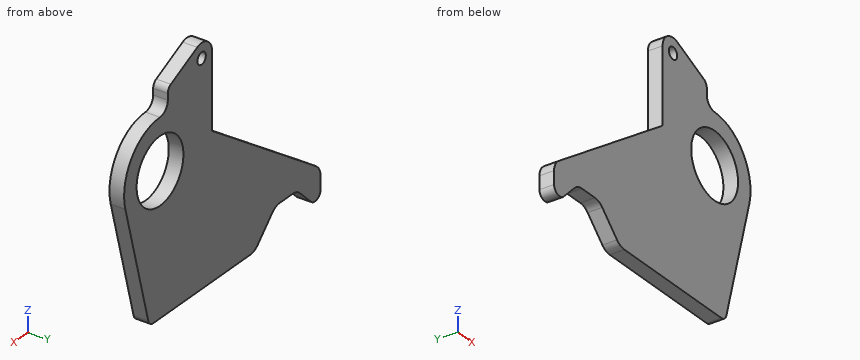
```python
from build123d import *

# Parameters (mm, degrees)
SKETCH1_R           = 2.5527
SKETCH1_R_2         = 14.2875
BOSS_EXTRUDE1_DEPTH = 6.35


with BuildPart() as part:
    # Sketch1 → Boss-Extrude1 (new body)
    with BuildSketch(Plane(origin=(0, 0, 0), x_dir=(1, 0, 0), z_dir=(0, 1, 0))):
        with BuildLine():
            Line((4.080014702, -3.175), (-55.087853576, -3.175))
            ThreePointArc((-55.087853576, -3.175), (-57.517893372, -3.658364969), (-59.577981637, -5.034871939))
            Line((-59.577981637, -5.034871939), (-68.558237758, -14.015128061))
            ThreePointArc((-68.558237758, -14.015128061), (-70.618326023, -15.391635031), (-73.048365818, -15.875))
            Line((-73.048365818, -15.875), (-80.939134182, -15.875))
            ThreePointArc((-80.939134182, -15.875), (-83.369173977, -15.391635031), (-85.429262242, -14.015128061))
            Line((-85.429262242, -14.015128061), (-92.164454333, -7.27993597))
            ThreePointArc((-92.164454333, -7.27993597), (-93.194498465, -6.591682484), (-94.409518363, -6.35))
            Line((-94.409518363, -6.35), (-94.77375, -6.35))
            ThreePointArc((-94.77375, -6.35), (-97.01881403, -7.27993597), (-97.94875, -9.525))
            Line((-97.94875, -9.525), (-97.94875, -15.200863174))
            ThreePointArc((-97.94875, -15.200863174), (-97.231268791, -18.132966868), (-95.240960371, -20.402478656))
            Line((-95.240960371, -20.402478656), (-31.75, -64.859327715))
            Line((-31.75, -64.859327715), (-31.75, -97.4852))
            ThreePointArc((-31.75, -97.4852), (-28.819730055, -102.835708981), (-22.733323984, -103.248127991))
            Line((-22.733323984, -103.248127991), (-6.604161992, -95.784691086))
            ThreePointArc((-6.604161992, -95.784691086), (-5.26224551, -94.613092118), (-4.7625, -92.903227091))
            Line((-4.7625, -92.903227091), (-4.7625, -90.17))
            ThreePointArc((-4.7625, -90.17), (-3.367596045, -86.802403955), (0, -85.4075))
            ThreePointArc((0, -85.4075), (17.380388302, -76.836441006), (21.161020039, -57.829921769))
            Line((21.161020039, -57.829921769), (7.146829201, -5.528249532))
            ThreePointArc((7.146829201, -5.528249532), (6.012832239, -3.831103145), (4.080014702, -3.175))
        make_face()
        with Locations((-25.4, -97.4852)):
            Circle(SKETCH1_R, mode=Mode.SUBTRACT)
        with Locations((0, -63.5)):
            Circle(SKETCH1_R_2, mode=Mode.SUBTRACT)
    extrude(amount=-BOSS_EXTRUDE1_DEPTH)


solid = part.part
```
The listing builds one solid part. Answer for the finished solid, in the listing's coordinates (mm). Round coordinates to 2 decimals unless told otherwise and drop trailing zeros. Order: outer loops, then holes, each group sorted by start corner. A loop starts at its lowest first (then second) coordinate and runs counter-clockwise, first axis right, second up. Notation, with made-up numbers: (22.25, 15.5) -> (31.25, 15.5) arc R16 cw to (31.25, 43.5) -> close; hole circle Ø6 at (-4, 1.5). An arc over 180 degrees is marked (long way). Answer as CSV lines item,"result".
Q1. A cutting plane is placed at D-D on z = 23. Determine the outline of the cut face in (x, y), plus the area to 3 significant figures.
Computed values:
outline,"(-91.53, -6.35) -> (11.83, -6.35) -> (11.83, 0) -> (-91.53, 0) -> close"
area,"656 mm^2"
Q2. A cutting plane is placed at B-B on y = -3.75. Give the number of separate pieces and of enclosed holes in the cut face, plus the area to 3 significant figures.
Computed values:
separate pieces,"1"
enclosed holes,"2"
area,"5,820 mm^2"
Q3. Consider line 1 (Z direction, x = -25.4, y = -2.5) (1 decimal); line 2 (X direction, y = -5.25, z = 92); line 3 (Z direction, x = -42, y = -0.25) (3 decimals). Determine where each line is inside the solid, lowest interval first. Write a range as from..to.
Computed values:
line 1,"z = 3.2..94.9, 100..103.8"
line 2,"x = -31.75..-4.76"
line 3,"z = 3.175..57.682"
Q4. A cutting plane is placed at C-C on z = 63.5. Determine the outline of the cut face in (x, y), plus the area to 3 significant figures.
Computed values:
outline,"(-33.69, -6.35) -> (-14.29, -6.35) -> (-14.29, 0) -> (-33.69, 0) -> close; (14.29, -6.35) -> (21.91, -6.35) -> (21.91, 0) -> (14.29, 0) -> close"
area,"172 mm^2"
Q5. Given pin 1 (10 mm diameter, centred on x = -36, z = 13.5, fed in from +Y); pin 2 (0.8 mm diameter, centred on y = -3, z = 92, fed in from +X); pin 3 (1.9 mm diameter, centred on y = -2, z = 80, fed in from -X); pin 4 (1.9 mm diameter, centred on x = -79, y = -2, fed in from -Z) (3 decimals), each flat-ended and moving along its own axis, determine where each tip first touches the part or whether it passes through.
Computed values:
pin 1,"stops at y = 0"
pin 2,"stops at x = -4.76"
pin 3,"stops at x = -31.75"
pin 4,"stops at z = 15.875"
